Source: three-view drawing plus pictorial views. Frame: mm from the lowest corner of the part. Round coordinates to 2 decimals unless told otherwise and drop trailing zeros. Write each loop counter-clockwise with the first axis right and the second up, starting at its lowest first coordinate (ties: lowest second). Pieces come first, ordered by that corner, then holes.
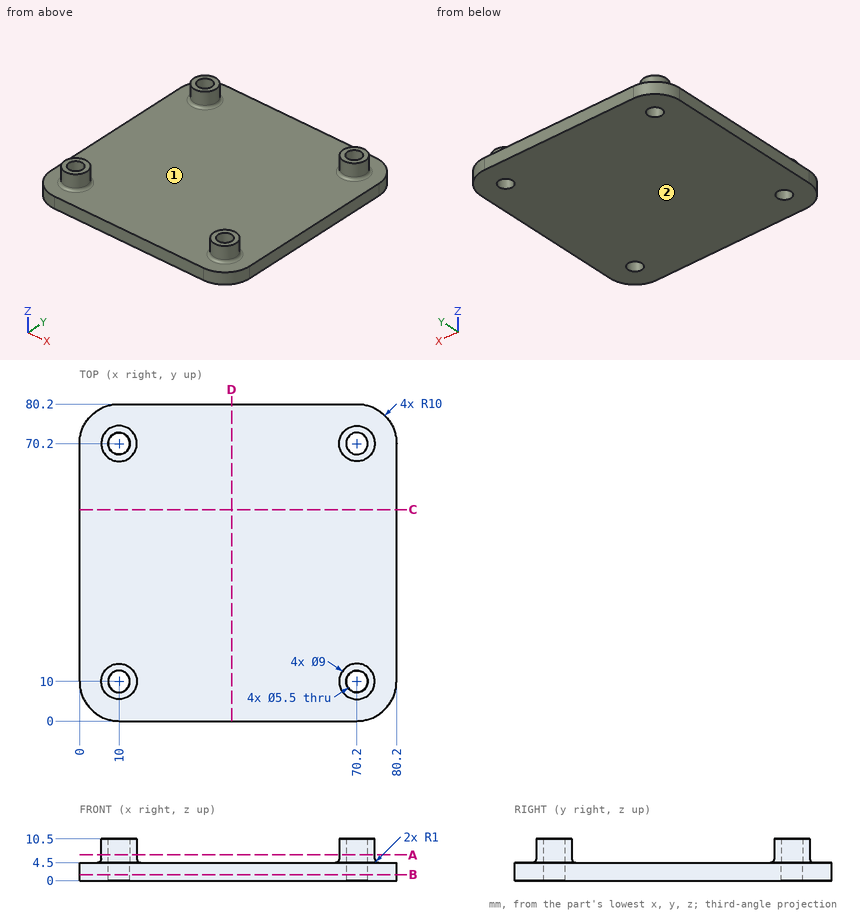
1) Draft query along X for the marked faces 1 and 2. Return one class per face: pulls with the +X half, pulls with the -X half, needs draft (parallel to the pull), parting line crosses it, or undercut.
2) Section C-C on y = 53.5. Output: boundary loops of the cut face in (x, z).
3) First-contact query: P1, Ø6, axis at x = 53, y = 58, coming from the +Z side; P2, Ø4.5, axis at x = 10, y = 70.2, coming from the -Z side. Flat tips, straight axial feed; report the tip coordinate or a pass-through.
4) Line query: probe 1 along Y at (x, z) = (10, 8); probe 2 along Y at (x, z) = (10, 1.4). Output: solid intervals per line, ascending.
5) Section A-A on z = 6.5. Output: boundary loops of the cut face in (x, y).
6) Section B-B on z = 1.5. Output: boundary loops of the cut face in (x, y), plus the area to 3 significant figures.
Filled in:
1. face 1: undercut
1. face 2: needs draft
2. outline: (0, 0) - (80.2, 0) - (80.2, 4.5) - (0, 4.5) - close
3. P1: stops at z = 4.5
3. P2: passes through
4. probe 1: y = 5.5 to 7.25, 12.75 to 14.5, 65.7 to 67.45, 72.95 to 74.7
4. probe 2: y = 0 to 7.25, 12.75 to 67.45, 72.95 to 80.2
5. outline: circle Ø9 at (10, 10); circle Ø9 at (10, 70.2); circle Ø9 at (70.2, 10); circle Ø9 at (70.2, 70.2); hole circle Ø5.5 at (10, 10); hole circle Ø5.5 at (10, 70.2); hole circle Ø5.5 at (70.2, 10); hole circle Ø5.5 at (70.2, 70.2)
6. outline: (0, 10) arc R10 ccw to (10, 0) - (70.2, 0) arc R10 ccw to (80.2, 10) - (80.2, 70.2) arc R10 ccw to (70.2, 80.2) - (10, 80.2) arc R10 ccw to (0, 70.2) - close; hole circle Ø5.5 at (10, 10); hole circle Ø5.5 at (10, 70.2); hole circle Ø5.5 at (70.2, 10); hole circle Ø5.5 at (70.2, 70.2)
6. area: 6,250 mm2
